from build123d import *

# Parameters (mm, degrees)
BOSS_EXTRUDE5_DEPTH   = 10
CUT_EXTRUDE6_DEPTH    = 5
FILLET4_R             = 1
FILLET4_OF_MIRROR25_R = 1


with BuildPart() as part:
    # Sketch15 → Boss-Extrude5 (new body)
    with BuildSketch(Plane(origin=(0, 0, 0), x_dir=(1, 0, 0), z_dir=(0, 1, 0))):
        Polygon((24.3, 76.900659127), (-6.625, 76.900659127), (-6.625, -4.5), (24.3, -4.5), (24.3, 44.900659127), (21.675, 44.900659127), (21.675, 47.400659127), (21.675, 72.400659127), (21.675, 74.900659127), (24.3, 74.900659127), align=None)
        Polygon((-2.625, 25), (-2.625, 0), (-2.625, -2.5), (0, -2.5), (2.625, -2.5), (2.625, 0), (2.625, 25), (2.625, 27.5), (0, 27.5), (-2.625, 27.5), align=None, mode=Mode.SUBTRACT)
    boss_extrude5 = extrude(amount=BOSS_EXTRUDE5_DEPTH)

    # Sketch18 → Cut-Extrude6 (cut)
    with BuildSketch(Plane(origin=(0, 10, 0), x_dir=(1, 0, 0), z_dir=(0, 1, 0))):
        Polygon((21.675, 51.3980649), (-4.44053483, 51.3980649), (-4.44053483, 20.8980649), (24.3, 20.8980649), (24.3, 51.3980649), align=None)
    cut_extrude6 = extrude(amount=-CUT_EXTRUDE6_DEPTH, mode=Mode.SUBTRACT)

    # Fillet4
    fillet4_edges = [part.edges().sort_by_distance(p)[0] for p in [
        (21.675, 5, -74.900659127),
        (-2.625, 5, 2.5),
        (2.625, 5, 2.5),
        (2.625, 2.5, -27.5),
        (-2.625, 2.5, -27.5),
        (21.675, 2.5, -44.900659127),
    ]]
    fillet(fillet4_edges, radius=FILLET4_R)

    # Mirror25: Boss-Extrude5, Cut-Extrude6 across plane
    add(boss_extrude5.mirror(Plane(origin=(24.3, 10, 4.5), x_dir=(0, 0, 1), z_dir=(-1, 0, 0))))
    add(cut_extrude6.mirror(Plane(origin=(24.3, 10, 4.5), x_dir=(0, 0, 1), z_dir=(-1, 0, 0))), mode=Mode.SUBTRACT)

    # Fillet4 of Mirror25
    fillet4_of_mirror25_edges = [part.edges().sort_by_distance(p)[0] for p in [
        (26.925, 5, -74.900659127),
        (51.225, 5, 2.5),
        (45.975, 5, 2.5),
        (45.975, 2.5, -27.5),
        (51.225, 2.5, -27.5),
        (26.925, 2.5, -44.900659127),
    ]]
    fillet(fillet4_of_mirror25_edges, radius=FILLET4_OF_MIRROR25_R)


solid = part.part
Geometry: final body of the model. Coordinates: model frame, mm. A direction names the side the tool comes from. Round coordinates to 2 decimals unless told otherwise and drop trailing zeros. Write each loop counter-clockwise with the first axis right and the second up, starting at its lowest first coordinate (ties: lowest second). Pieces come first, ordered by that corner, then holes. Notation, with made-up numbers: M -1,63 L 28,63 A23 ccw 28,102 Z; hole C 10,-23.75 d11. An arc over 180 degrees is marked long. Write item = value, one per line.
Item 1: Section query A-A on z = -67.5. Return loops of the section in (x, y) (3 decimals).
Findings:
outline = M -6.625,0 L 21.675,0 L 21.675,10 L -6.625,10 Z; M 26.925,0 L 55.225,0 L 55.225,10 L 26.925,10 Z
Item 2: Section query B-B on y = 1.25. Return loops of the section in (x, z) (3 decimals), then the cut area to 3 significant figures.
Findings:
outline = M -6.625,-76.901 L 55.225,-76.901 L 55.225,4.5 L -6.625,4.5 Z; hole M -2.625,-26.5 A1 ccw -1.625,-27.5 L 1.625,-27.5 A1 ccw 2.625,-26.5 L 2.625,1.5 A1 ccw 1.625,2.5 L -1.625,2.5 A1 ccw -2.625,1.5 Z; hole M 21.675,-73.901 A1 ccw 22.675,-74.901 L 25.925,-74.901 A1 ccw 26.925,-73.901 L 26.925,-45.901 A1 ccw 25.925,-44.901 L 22.675,-44.901 A1 ccw 21.675,-45.901 Z; hole M 45.975,-26.5 A1 ccw 46.975,-27.5 L 50.225,-27.5 A1 ccw 51.225,-26.5 L 51.225,1.5 A1 ccw 50.225,2.5 L 46.975,2.5 A1 ccw 45.975,1.5 Z
area = 4,560 mm^2
Item 3: Section query D-D on y = 6.5. Return loops of the section in (x, z) (3 decimals).
Findings:
outline = M -6.625,-76.901 L 55.225,-76.901 L 55.225,4.5 L -6.625,4.5 Z; hole M -4.441,-51.398 L 21.675,-51.398 L 21.675,-73.901 A1 ccw 22.675,-74.901 L 25.925,-74.901 A1 ccw 26.925,-73.901 L 26.925,-51.398 L 53.041,-51.398 L 53.041,-20.898 L 51.225,-20.898 L 51.225,1.5 A1 ccw 50.225,2.5 L 46.975,2.5 A1 ccw 45.975,1.5 L 45.975,-20.898 L 2.625,-20.898 L 2.625,1.5 A1 ccw 1.625,2.5 L -1.625,2.5 A1 ccw -2.625,1.5 L -2.625,-20.898 L -4.441,-20.898 Z
Item 4: Pin query (flat end, axial travel): P1, Ø15, axis at x = 37, z = -42, coming from the +Y side. Return the tip coordinate at first contact, or that it passes through.
Findings:
P1 = 5
Item 5: Section query C-C on z = -12. Return loops of the section in (x, y) (3 decimals).
Findings:
outline = M -6.625,0 L -2.625,0 L -2.625,10 L -6.625,10 Z; M 2.625,0 L 45.975,0 L 45.975,10 L 2.625,10 Z; M 51.225,0 L 55.225,0 L 55.225,10 L 51.225,10 Z
Item 6: Pull-direction query (X, two-part tool) for faces 1 (the face through (-6.625, 5, -37)), 2 (the face through (24, 2, -44.901)), 3 (the face through (25, 0, -37)); classes: pulls with the +X half, pulls with the -X half, needs draft (parallel to the pull), parting line crosses it, or undercut.
Findings:
face_1 = pulls with the -X half
face_2 = undercut
face_3 = needs draft
Item 7: Access query for faces 4 (the face through (0, 2, -27.5)), 5 (the face through (-4, 8, -20.898)), 6 (the face through (24, 5, -76.901)). Directions: +Z, -Z, +X, -X, +Y, -Y. A direction counts if a zero-diameter tool reaches every point of the face in a straight line with its end or side. Return the directions, or none.
Findings:
face_4 = +Y, -Y
face_5 = +Y
face_6 = -Z, +X, -X, +Y, -Y
Item 8: Material intervals for line 1 along X through (y, z) = (3.25, -24) (3 decimals); line 2 along Z through (x, y) = (5.5, 7.5); line 3 along X through (y, z) = (4.75, -62.5) (3 decimals), sorted ascending. Write a range as [from, to].
Findings:
line_1 = [-6.625, -2.625], [2.625, 45.975], [51.225, 55.225]
line_2 = [-76.9, -51.4], [-20.9, 4.5]
line_3 = [-6.625, 21.675], [26.925, 55.225]
